from build123d import *

# Parameters (mm, degrees)
EXTRUDE_1_DEPTH     = 0.3
SKETCH_2_R          = 0.398831964
CUT_EXTRUDE_1_DEPTH = 10


with BuildPart() as part:
    # 草图1 → 凸台-拉伸1 (new body)
    with BuildSketch(Plane(origin=(0, 0, 3.15), x_dir=(-1, 0, 0), z_dir=(0, 0, -1))):
        with BuildLine():
            Line((-2.85, -3), (2.85, -3))
            ThreePointArc((2.85, -3), (2.956066017, -2.956066017), (3, -2.85))
            Line((3, -2.85), (3, 2.85))
            ThreePointArc((3, 2.85), (2.956066017, 2.956066017), (2.85, 3))
            Line((2.85, 3), (-2.85, 3))
            ThreePointArc((-2.85, 3), (-2.956066017, 2.956066017), (-3, 2.85))
            Line((-3, 2.85), (-3, -2.85))
            ThreePointArc((-3, -2.85), (-2.956066017, -2.956066017), (-2.85, -3))
        make_face()
    extrude(amount=-EXTRUDE_1_DEPTH)

    # 草图2 → 切除-拉伸1 (cut)
    with BuildSketch(Plane.XY.offset(3.45)):
        Circle(SKETCH_2_R)
    extrude(amount=-CUT_EXTRUDE_1_DEPTH, mode=Mode.SUBTRACT)


solid = part.part
Build history of the part. All positions in model axes, mm. Round coordinates to 2 decimals unless told otherwise and drop trailing zeros. Write each loop counter-clockwise with the first axis right and the second up, starting at its lowest first coordinate (ties: lowest second). Pieces come first, ordered by that corner, then holes. Notation, with made-up numbers: (-3, 76.25) - (39, 76.25) arc R20 cw to (39, 115.25) - close; hole circle Ø2 at (75, 70.25). An arc over 180 degrees is marked (long way). Use CSV: the item, a comma, the result in double quotes.
(1) Wall check: line 1 (Y direction, x = 0, z = 3.35). Give the ranges that are in metal, low to high.
Response:
line 1,"-3 to -0.4, 0.4 to 3"
(2) Band-saw the part on A-A (x = 0). Write the cut outline in (y, z), plus the area to 3 significant figures.
Response:
outline,"(-3, 3.15) - (-0.4, 3.15) - (-0.4, 3.45) - (-3, 3.45) - close; (0.4, 3.15) - (3, 3.15) - (3, 3.45) - (0.4, 3.45) - close"
area,"1.56 mm²"
